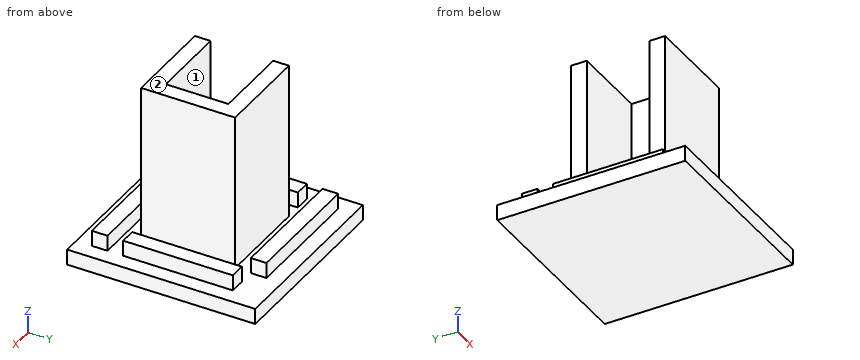
from build123d import *

# Parameters (mm, degrees)
F0_W     = 60
F0_H     = 60
F1_DEPTH = 5
F2_W     = 40
F2_H     = 5
F2_W_2   = 5
F2_H_2   = 35
F3_DEPTH = 5
F4_W     = 25
F4_H     = 5
F5_DEPTH = 50


with BuildPart() as f1:
    # F0 (on Top) → F1 (new body)
    with BuildSketch(Plane.XY):
        with Locations((30, 30)):
            Rectangle(F0_W, F0_H)
    extrude(amount=F1_DEPTH)

    # F2 (on face) → F3 (join)
    with BuildSketch(Plane.XY.offset(5)):
        with Locations((35, 7.5)):
            Rectangle(F2_W, F2_H)
        with Locations((52.5, 32.5)):
            Rectangle(F2_W_2, F2_H_2)
        with Locations((25, 52.5)):
            Rectangle(F2_W, F2_H)
        with Locations((7.5, 27.5)):
            Rectangle(F2_W_2, F2_H_2)
    extrude(amount=F3_DEPTH)

    # F4 (on face) → F5 (join)
    with BuildSketch(Plane.XY.offset(5)):
        Polygon((45, 45), (40, 45), (40, 40), (40, 20), (40, 15), (45, 15), align=None)
        with Locations((27.5, 42.5)):
            Rectangle(F4_W, F4_H)
        with Locations((27.5, 17.5)):
            Rectangle(F4_W, F4_H)
    extrude(amount=F5_DEPTH)


solid = f1.part
For this review, take the finished solid that the model builds, in its own axes (mm). Face numbers are marked on the shaded views. Give positions to 0.01 mm unless a question says otherwise; leave off trailing zeros. Loops run counter-clockwise (first coordinate to the right, second up) from the corner with the lowest first, then second, coordinate; pieces in that order, holes last. Notation, with made-up numbers: (-1, 26.5) -> (19, 26.5) arc R19 ccw to (19, 57.5) -> close; hole circle Ø8 at (87.25, -20.75). An arc over 180 degrees is marked (long way). One line per question, with ' | ' between items.
1) We need section D-D (x = 23). Write out the cut boundary in (y, z).
Resolved:
outline: (0, 0) -> (60, 0) -> (60, 5) -> (55, 5) -> (55, 10) -> (50, 10) -> (50, 5) -> (45, 5) -> (45, 55) -> (40, 55) -> (40, 5) -> (20, 5) -> (20, 55) -> (15, 55) -> (15, 5) -> (10, 5) -> (10, 10) -> (5, 10) -> (5, 5) -> (0, 5) -> close
2) The part is to be moulded in two halves that separate along Y. For the marked faces 1 and 2, say which applies: +Y half, -Y half, draft (parallel to the pull), parting line (faces both ways), or undercut.
Resolved:
face 1: undercut | face 2: draft
3) We need section B-B (x = 13). Write out the cut boundary in (y, z), plus the area to 3 significant figures.
Resolved:
outline: (0, 0) -> (60, 0) -> (60, 5) -> (55, 5) -> (55, 10) -> (50, 10) -> (50, 5) -> (0, 5) -> close | area: 325 mm2
4) We need section C-C (y = 33). Write out the cut boundary in (x, z), plus the area to 3 significant figures.
Resolved:
outline: (0, 0) -> (60, 0) -> (60, 5) -> (55, 5) -> (55, 10) -> (50, 10) -> (50, 5) -> (45, 5) -> (45, 55) -> (40, 55) -> (40, 5) -> (10, 5) -> (10, 10) -> (5, 10) -> (5, 5) -> (0, 5) -> close | area: 600 mm2
5) To check wall thickness, follow probe 1 along Y at (x, z) = (30, 7); probe 2 along Y at (x, z) = (22, 30.5); probe 3 along Z at (x, y) = (57, 12). State the ranges of each line that lie inside material, in increasing order.
Resolved:
probe 1: y = 5 to 10, 15 to 20, 40 to 45, 50 to 55 | probe 2: y = 15 to 20, 40 to 45 | probe 3: z = 0 to 5
6) We need section A-A (y = 6). Write out the cut boundary in (x, z), plus the area to 3 significant figures.
Resolved:
outline: (0, 0) -> (60, 0) -> (60, 5) -> (55, 5) -> (55, 10) -> (15, 10) -> (15, 5) -> (0, 5) -> close | area: 500 mm2
7) Insertion check: pin 1 Ø2.5 at (y, z) = (33, 7) entering from +X; pin 2 Ø5.5 at (y, z) = (17.5, 28.5) entering from -X; pin 3 Ø1.5 at (y, z) = (52, 7.5) entering from -X. Each pin has a flat end and moves straight along its axis. Give the tip position at first contact, or say it passes through.
Resolved:
pin 1: stops at x = 55 | pin 2: stops at x = 15 | pin 3: stops at x = 5
